from build123d import *

# Parameters (mm, degrees)
SKETCH2_R                      = 70
BOSS_EXTRUDE1_DEPTH            = 15
SKETCH5_R                      = 30.9
CUT_EXTRUDE1_DEPTH             = 12
SKETCH6_R                      = 28.8
CUT_EXTRUDE2_DEPTH             = 100.719606899
FILLET1_R                      = 2
CBORE_FOR_M5_SHCS1_D           = 5.5
CBORE_FOR_M5_SHCS1_CBORE_D     = 10
CBORE_FOR_M5_SHCS1_CBORE_DEPTH = 5


with BuildPart() as part:
    # Sketch2 → Boss-Extrude1 (new body)
    with BuildSketch(Plane(origin=(0, 0, 0), x_dir=(1, 0, 0), z_dir=(0, 1, 0))):
        with Locations(Location((0, 0, 0), (0, 0, 270))):
            Circle(SKETCH2_R)
    extrude(amount=BOSS_EXTRUDE1_DEPTH)

    # Sketch5 → Cut-Extrude1 (cut)
    with BuildSketch(Plane(origin=(0, 15, 0), x_dir=(1, 0, 0), z_dir=(0, 1, 0))):
        with Locations(Location((0, 0, 0), (0, 0, 270))):
            Circle(SKETCH5_R)
    extrude(amount=-CUT_EXTRUDE1_DEPTH, mode=Mode.SUBTRACT)

    # Sketch6 → Cut-Extrude2 (cut, through all)
    with BuildSketch(Plane(origin=(0, 3, 0), x_dir=(1, 0, 0), z_dir=(0, 1, 0))):
        with Locations(Location((0, 0, 0), (0, 0, 270))):
            Circle(SKETCH6_R)
    extrude(amount=-CUT_EXTRUDE2_DEPTH, mode=Mode.SUBTRACT)

    # Fillet1
    fillet1_edges = [part.edges().sort_by_distance(p)[0] for p in [
        (0, 0, -70),
        (0, 15, -70),
        (0, 15, -30.9),
    ]]
    fillet(fillet1_edges, radius=FILLET1_R)

    # CBORE for M5 SHCS1 (through all)
    with Locations(Plane(origin=(0, 15, 0), x_dir=(1, 0, 0), z_dir=(0, 1, 0))):
        with Locations((0, 60), (60, 0), (-60, 0), (0, -60)):
            CounterBoreHole(CBORE_FOR_M5_SHCS1_D / 2, CBORE_FOR_M5_SHCS1_CBORE_D / 2, CBORE_FOR_M5_SHCS1_CBORE_DEPTH)


solid = part.part
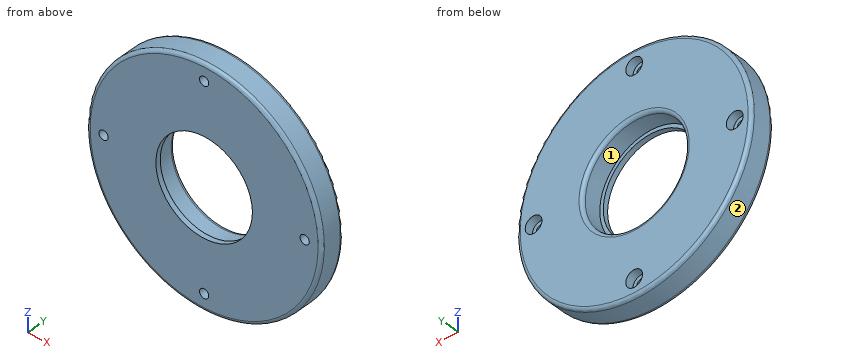
CAD build for the part. Positions are in the model's coordinates, mm. Face numbers are marked on the shaded views. A direction names the side the tool comes from. Coordinates: 2 decimals unless noted, no trailing zeros. Write each loop counter-clockwise with the first axis right and the second up, starting at its lowest first coordinate (ties: lowest second). Pieces come first, ordered by that corner, then holes. Notation, with made-up numbers: (61.25, 81.25) - (84.25, 81.25) arc R12 cw to (84.25, 96.25) - close; hole circle Ø10 at (5, 68). An arc over 180 degrees is marked (long way). Use a Markdown table: item, result. Add a question column.
Item 1: Band-saw the part on C-C, the plane y = 8. Give the cut face in (x, z), and give its area (3 significant figures).
Item 2: Flat gauge pins, fed straight in: pin 1 (11.5 mm diameter, centred on x = 0, z = 60, fed in from -Y); pin 2 (5 mm diameter, centred on x = 49.5, y = 13, fed in from -Z); pin 3 (5 mm diameter, centred on x = -0.5, z = 62, fed in from +Y); pin 4 (3.5 mm diameter, centred on x = 0, z = -60, fed in from -Y). Where does each tip first touch, or does it go through?
Item 3: Drill centre lines: L1, parallel to Z at x = 2, y = 14; L2, parallel to X at y = 11, z = 2; L3, parallel to X at y = 13.9, z = 60. Where is each one in solid material? Low to high. Write a range as from..to.
Item 4: 3-axis set-ups, long thin cutter, end or side, ignore diameter. For the marked faces 1 and 2: which of +Z, -Z, +X, -X, +Y, -Y reach the whole face in a straight line?
Item 5: Band-saw the part on A-A, the plane z = 0. Give the number of separate pieces and of enclosed holes in the cut face, and give its area (3 significant figures).
Numbers:
| question | item | result |
|---|---|---|
| 1 | outline | circle Ø140 at (0, 0); hole circle Ø5.5 at (-60, 0); hole circle Ø61.8 at (0, 0); hole circle Ø5.5 at (0, -60); hole circle Ø5.5 at (0, 60); hole circle Ø5.5 at (60, 0) |
| 1 | area | 12,300 mm2 |
| 2 | pin 1 | y = 0 |
| 2 | pin 2 | z = -51.87 |
| 2 | pin 3 | y = 10 |
| 2 | pin 4 | through |
| 3 | L1 | -69.7..-64.58, -55.42..-31.1, 31.1..55.42, 64.58..69.7 |
| 3 | L2 | -69.97..-64.58, -55.42..-30.84, 30.84..55.42, 64.58..69.97 |
| 3 | L3 | -35.64..-5, 5..35.64 |
| 4 | face 1 | +Y |
| 4 | face 2 | +Y, -Y |
| 5 | separate pieces | 4 |
| 5 | enclosed holes | 0 |
| 5 | area | 970 mm2 |
